For this review, take the finished solid that the model builds, in its own axes (mm). Face numbers are marked on the shaded views. A direction names the side the tool comes from. Coordinates: 2 decimals unless noted, no trailing zeros. Order: outer loops, then holes, each group sorted by start corner. A loop starts at its lowest first (then second) coordinate and runs counter-clockwise, first axis right, second up. Notation, with made-up numbers: (68, 38.5) - (124, 38.5) arc R19 ccw to (124, 46.5) - close; hole circle Ø11 at (72, 37). An arc over 180 degrees is marked (long way). One line per item, written item: value. Start each with the question number.
(1) Clearance check with flat-ended pins moving along their axes: pin 1 (2.5 mm diameter, centred on x = 4, z = 3, fed in from +Y); pin 2 (1.1 mm diameter, centred on x = 0, z = 5, fed in from +Y); pin 3 (1.5 mm diameter, centred on x = 10.5, z = 10.5, fed in from +Y); pin 4 (10 mm diameter, centred on y = 31.5, z = 4, fed in from +X). State where each tip first meets the part, or that it passes through.
(2) Consider section B-B on x = 7.75. Write out the cut boundary in (y, z), then the cut area to 3 significant figures.
(3) To check wall thickness, follow line 1 along Z through (x, y) = (0, 13.25); line 2 along X through (y, z) = (20.5, -0.25); line 3 along Z through (x, y) = (0, 3.2). State the ranges of each line that lie inside material, in increasing order.
(4) Consider section C-C on y = 4. Write out the cut boundary in (x, z), then the cut area to 3 significant figures.
(5) For the marked faces 1, 2 and 3, list the 3-axis set-ups (+Z, -Z, +X, -X, +Y, -Y) from which the entire face can be reached by the end or side of a thin tool; tool diameter is ignored.
(6) Consider section A-A on z = 8.5. Write out the cut boundary in (x, y).
(7) Consider section D-D on y = 22. Write out the cut boundary in (x, z), then the cut area to 3 significant figures.
(8) Mouldability with a two-part tool opening along Z and no side actions: class the marked faces 4, 5 and 6 as released by +Z, released by -Z, zero draft, split by the parting line, or undercut.
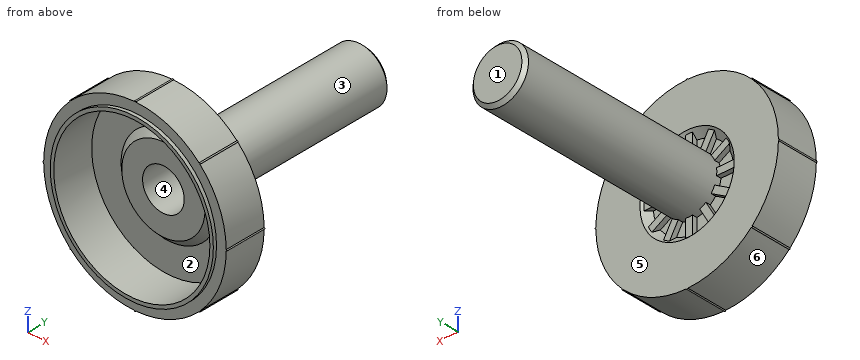
Autodesk Inventor part; units mm, degrees
ref_plane "YZ Plane" through (0, 0, 0) normal (1, 0, 0) x (0, 1, 0)
ref_plane "XZ Plane" through (0, 0, 0) normal (0, 1, 0) x (-1, 0, 0)
ref_plane "XY Plane" through (0, 0, 0) normal (0, 0, 1) x (1, 0, 0)
sketch "Sketch1" plane through (0, 0, 0) normal (0, 1, 0) x (-1, 0, 0)
  circle A0 centre (0, 0) radius 13.15
  dimension "d0" = 26.3
extrude "Extrusion1" add sketch "Sketch1" along normal blind 6.5
sketch "Sketch2" plane through (0, 0, 0) normal (0, -1, 0) x (1, 0, 0)
  circle A0 centre (0, 0) radius 13.15
  circle A1 centre (0, 0) radius 11.75
  dimension "d3" = 23.5
extrude "Extrusion2" cut sketch "Sketch2" against normal blind 0.5
sketch "Sketch3" plane through (0, 0, 0) normal (0, -1, 0) x (1, 0, 0)
  circle A0 centre (0, 0) radius 11.25
  dimension "d6" = 22.5
extrude "Extrusion3" cut sketch "Sketch3" against normal blind 6
sketch "Sketch4" plane through (0, 6.5, 0) normal (0, 1, 0) x (1, 0, 0)
  circle A0 centre (0, 0) radius 4
  dimension "d9" = 8
extrude "Extrusion4" add sketch "Sketch4" along normal blind 30
chamfer "Chamfer1" distance 0.5 angle 45 1 edges at (-4, 36.5, 0)
sketch "Sketch5" plane through (0, 6, 0) normal (0, -1, 0) x (1, 0, 0)
  circle A0 centre (0, 0) radius 7
  dimension "d15" = 14
extrude "Extrusion5" add sketch "Sketch5" along normal blind 1
chamfer "Chamfer2" distance 1 angle 45 1 edges at (-7, 5, 0)
sketch "Sketch6" plane through (0, 5, 0) normal (0, -1, 0) x (1, 0, 0)
  point P0 (0, 0)
hole "Hole1" at (0, 5, 0) direction (0, 1, 0) diameter 6 depth 30
sketch "Sketch7" plane through (0, 0, 0) normal (1, 0, 0) x (0, 1, 0)
  line L0 (6.5, 4) -> (6.5, -4)
  line L1 (6.5, -4) -> (5.5, -4)
  line L2 (5.5, -4) -> (5.5, -5.7929)
  line L3 (5.5, -5.7929) -> (6.5, -6.7929)
  line L4 (6.5, -13.15) -> (6.5, 13.15)
  line L5 (0.5, -11.75) -> (0, -11.75)
  line L6 (0, -11.75) -> (0, -11.25)
  line L7 (0, -11.25) -> (6, -11.25)
  line L8 (6, -11.25) -> (6, -7)
  line L9 (6, -7) -> (5, -6)
  line L10 (5, -6) -> (5, -3)
  line L11 (5, -3) -> (35, -3)
  line L12 (35, -3) -> (35, 3)
  line L13 (35, 3) -> (5, 3)
  line L14 (5, 3) -> (5, 6)
  line L15 (5, 6) -> (6, 7)
  line L16 (6, 7) -> (6, 11.25)
  line L17 (6, 11.25) -> (0, 11.25)
  line L18 (0, 11.25) -> (0, 11.75)
  line L19 (0, 11.75) -> (0.5, 11.75)
  line L20 (0.5, 11.75) -> (0.5, 13.15)
  line L21 (0.5, 13.15) -> (6.5, 13.15)
  line L22 (6.5, 13.15) -> (6.5, 4)
  line L23 (6.5, 4) -> (36, 4)
  line L24 (36, 4) -> (36.5, 3.5)
  line L25 (36.5, 3.5) -> (36.5, -3.5)
  line L26 (36.5, -3.5) -> (36, -4)
  line L27 (36, -4) -> (6.5, -4)
  line L28 (6.5, -4) -> (6.5, -13.15)
  line L29 (6.5, -13.15) -> (0.5, -13.15)
  line L30 (0.5, -13.15) -> (0.5, -11.75)
  line L31 (0, 0) -> (40, 0)
  dimension "d28" = 0.5
  dimension "d29" = 0.5
  dimension "d30" = 0.5
revolve "Revolution1" cut sketch "Sketch7" angle 360 about axis through (0, 0, 0) along (0, 1, 0) contours L4 L3 L2 L1
sketch "Sketch8" plane through (0, 0, 0) normal (1, 0, 0) x (0, 1, 0)
  line L0 (0.5, -11.75) -> (0, -11.75)
  line L1 (0, -11.75) -> (0, -11.25)
  line L2 (0, -11.25) -> (6, -11.25)
  line L3 (6, -11.25) -> (6, -7)
  line L4 (6, -7) -> (5, -6)
  line L5 (5, -6) -> (5, -3)
  line L6 (5, -3) -> (35, -3)
  line L7 (35, -3) -> (35, 3)
  line L8 (35, 3) -> (5, 3)
  line L9 (5, 3) -> (5, 6)
  line L10 (5, 6) -> (6, 7)
  line L11 (6, 7) -> (6, 11.25)
  line L12 (6, 11.25) -> (0, 11.25)
  line L13 (0, 11.25) -> (0, 11.75)
  line L14 (0, 11.75) -> (0.5, 11.75)
  line L15 (0.5, 11.75) -> (0.5, 13.15)
  line L16 (0.5, 13.15) -> (6.5, 13.15)
  line L17 (6.5, 13.15) -> (6.5, 6.7929)
  line L18 (6.5, 6.7929) -> (5.5, 5.7929)
  line L19 (5.5, 5.7929) -> (5.5, 4)
  line L20 (5.5, 4) -> (36, 4)
  line L21 (36, 4) -> (36.5, 3.5)
  line L22 (36.5, 3.5) -> (36.5, -3.5)
  line L23 (36.5, -3.5) -> (36, -4)
  line L24 (36, -4) -> (5.5, -4)
  line L25 (5.5, -4) -> (5.5, -5.7929)
  line L26 (5.5, -5.7929) -> (6.5, -6.7929)
  line L27 (6.5, -6.7929) -> (6.5, -13.15)
  line L28 (6.5, -13.15) -> (0.5, -13.15)
  line L29 (0.5, -13.15) -> (0.5, -11.75)
  line L30 (5.5, -3.5) -> (6.2, -3.5)
  line L31 (6.2, -3.5) -> (6.2, -6.4929)
  line L32 (6.2, -6.4929) -> (5.5, -6.4929)
  line L33 (5.5, -6.4929) -> (5.5, -3.5)
  line L34 (6.5, 6.7929) -> (6.5, -6.7929)
  point P0 (0, 0)
  point P1 (5.5, -4)
  dimension "d32" = 0.3
extrude "Extrusion6" add sketch "Sketch8" along normal mid plane 1 contours L26 L25 L24 L31 | L24 L33 L30 L31
pattern_circular "Circular Pattern1" count 12 over 360 about axis through (0, 6.5, 0) along (0, 1, 0) of "Extrusion6"
sketch "Sketch9" plane through (0, 6.5, 0) normal (0, 1, 0) x (1, 0, 0)
  line L0 (0, 0) -> (0, 13.8998)
  circle A0 centre (0, 0) radius 13.25
  circle A1 centre (0, 0) radius 6.7929
  circle A2 centre (0, 0) radius 4
  circle A3 centre (0, 0) radius 3
  circle A4 centre (0, 0) radius 13.15
  circle A5 centre (0, 13.15) radius 0.1
  dimension "d38" = 26.5
extrude "Extrusion7" add sketch "Sketch9" against normal up to surface (6 mm away) contours A5 A4 L0 | L0 A4 A5 | A4 A5 L0 | L0 A5 A4
pattern_circular "Circular Pattern2" count 8 over 360 about axis through (0, 6.5, 0) along (0, 1, 0) of "Extrusion7"
equation "\"d29\" = d28"
equation "\"d30\" = d28"
properties part number "Piston" material "Acetal Resin, White"
Geometry check:
1. pin 1: stops at y = 36.25
1. pin 2: stops at y = 6.2
1. pin 3: passes through
1. pin 4: stops at x = 4
2. outline: (0, -8.83) - (0.5, -8.83) - (0.5, -10.62) - (6.5, -10.62) - (6.5, 10.62) - (0.5, 10.62) - (0.5, 8.83) - (0, 8.83) - (0, 8.15) - (6, 8.15) - (6, -8.15) - (0, -8.15) - close
2. area: 38.5 mm^2
3. line 1: z = -4 to -3, 3 to 4
3. line 2: x = -3.99 to -2.99, 2.99 to 3.99
3. line 3: z = -13.25 to -11.25, 11.25 to 13.25
4. outline: (-13.15, -0.1) arc R13.15 ccw to (-9.37, -9.23) arc R0.1 ccw to (-9.23, -9.37) arc R13.15 ccw to (-0.1, -13.15) arc R0.1 ccw to (0.1, -13.15) arc R13.15 ccw to (9.23, -9.37) arc R0.1 ccw to (9.37, -9.23) arc R13.15 ccw to (13.15, -0.1) arc R0.1 ccw to (13.15, 0.1) arc R13.15 ccw to (9.37, 9.23) arc R0.1 ccw to (9.23, 9.37) arc R13.15 ccw to (0.1, 13.15) arc R0.1 ccw to (-0.1, 13.15) arc R13.15 ccw to (-9.23, 9.37) arc R0.1 ccw to (-9.37, 9.23) arc R13.15 ccw to (-13.15, 0.1) arc R0.1 ccw to start; hole circle Ø22.5 at (0, 0)
4. area: 146 mm^2
5. face 1: +Z, -Z, +X, -X, +Y
5. face 2: -Y
5. face 3: +Y
6. outline: (-10.03, 0.5) - (-8.11, 0.5) - (-8.11, 0) - (-7.37, 0) - (-7.37, 6) - (7.37, 6) - (7.37, 0) - (8.11, 0) - (8.11, 0.5) - (10.03, 0.5) - (10.03, 6.5) - (-10.03, 6.5) - close
7. outline: circle Ø8 at (0, 0); hole circle Ø6 at (0, 0)
7. area: 22.0 mm^2
8. face 4: undercut
8. face 5: zero draft
8. face 6: released by -Z
